Input: part model. Units: mm. Frame: model coordinates. A direction names the side the tool comes from. Round coordinates to 2 decimals unless told otherwise and drop trailing zeros. Loops run counter-clockwise (first coordinate to the right, second up) from the corner with the lowest first, then second, coordinate; pieces in that order, holes last.
(1) Cut plane B-B, the plane z = -8.5. Output: boundary loops of the cut face in (x, y), and give its area (3 significant figures).
(2) Line query: line 1 (Z direction, x = 4.15, y = 0); line 2 (Y direction, x = 4.2, z = -8.5); line 3 (Z direction, x = 3.25, y = 1). Output: solid intervals per line, ascending.
(3) Cut plane A-A, the plane x = -3.25. Output: boundary loops of the cut face in (y, z).
(4) First-contact query: pin 1 Ø6 at (x, y) = (3, -8) entering from -Z; pin 2 Ø1.5 at (x, y) = (0, 0.5) entering from +Z; pin 3 Ø4 at (y, z) = (-33.5, -1) entering from -X; pin 4 Ø1 at (y, z) = (-41, 4.5) entering from +X. Flat tips, straight axial feed; report the tip coordinate or a pass-through.
(5) Cut plane D-D, the plane z = 0. Output: boundary loops of the cut face in (x, y).
(6) Access query for faces 1 (the face through (-1, -3.5, -2.5)), 2 (the face through (5, 0, 0)), 3 (the face through (1.5, -2, 9)). Directions: +Z, -Z, +X, -X, +Y, -Y. A direction counts if a zero-diameter tool reaches every point of the face in a straight line with its end or side. Return the directions, or none.
(7) Cut plane C-C, the plane y = 0. Output: boundary loops of the cut face in (x, z), and give its area (3 significant figures).
(8) Draft query along X for faces 4 (the face through (-5, 0, 0)), 5 (the face through (-1.5, -2, -8)), 6 (the face through (3.27, -2.93, 11.9)). Return one class per face: released by +X, released by -X, zero draft, split by the parting line, or undercut.
from build123d import *

# Parameters (mm, degrees)
CROQUIS1_R                 = 2.5
SALIENTE_EXTRUIR1_DEPTH    = 50
CROQUIS2_R                 = 1.5
SALIENTE_EXTRUIR2_DEPTH    = 5
CORTAR_EXTRUIR1_DEPTH      = 56.167925464
CORTAR_EXTRUIR1_DEPTH_BACK = 56.167925464
CROQUIS3_W                 = 3
CROQUIS3_H                 = 8


with BuildPart() as part:
    # Croquis1 → Saliente-Extruir1 (new body)
    with BuildSketch(Plane(origin=(0, 0, 0), x_dir=(1, 0, 0), z_dir=(0, 1, 0))):
        with Locations(Location((0, 0, 0), (0, 0, 270))):
            Circle(CROQUIS1_R)
    extrude(amount=-SALIENTE_EXTRUIR1_DEPTH)

    # Croquis2 → Saliente-Extruir2 (add, symmetric)
    with BuildSketch(Plane(origin=(0, 0, 0), x_dir=(0, 0, -1), z_dir=(1, 0, 0))):
        with BuildLine():
            Line((10.5, -3.5), (-10.5, -3.5))
            ThreePointArc((-10.5, -3.5), (-11.914213562, -2.914213562), (-12.5, -1.5))
            Line((-12.5, -1.5), (-12.5, 1.5))
            ThreePointArc((-12.5, 1.5), (-11.914213562, 2.914213562), (-10.5, 3.5))
            Line((-10.5, 3.5), (10.5, 3.5))
            ThreePointArc((10.5, 3.5), (11.914213562, 2.914213562), (12.5, 1.5))
            Line((12.5, 1.5), (12.5, -1.5))
            ThreePointArc((12.5, -1.5), (11.914213562, -2.914213562), (10.5, -3.5))
        make_face()
        with Locations((-8.5, 0)):
            Circle(CROQUIS2_R, mode=Mode.SUBTRACT)
        with Locations((8.5, 0)):
            Circle(CROQUIS2_R, mode=Mode.SUBTRACT)
    extrude(amount=SALIENTE_EXTRUIR2_DEPTH, both=True)

    # Croquis3 → Cortar-Extruir1 (cut, two sides: drawn at the far end of the back side and taken through both)
    with BuildSketch(Plane(origin=(0, 3.5, 0), x_dir=(1, 0, 0), z_dir=(0, 1, 0)).offset(-CORTAR_EXTRUIR1_DEPTH_BACK)):
        with Locations((0, 8.5)):
            Rectangle(CROQUIS3_W, CROQUIS3_H)
        with Locations((0, -8.5)):
            Rectangle(CROQUIS3_W, CROQUIS3_H)
    extrude(amount=CORTAR_EXTRUIR1_DEPTH + CORTAR_EXTRUIR1_DEPTH_BACK, mode=Mode.SUBTRACT)


solid = part.part
Reported:
1. outline: (-5, -3.5) - (-1.5, -3.5) - (-1.5, -1.5) - (-5, -1.5) - close; (-5, 1.5) - (-1.5, 1.5) - (-1.5, 3.5) - (-5, 3.5) - close; (1.5, -3.5) - (5, -3.5) - (5, -1.5) - (1.5, -1.5) - close; (1.5, 1.5) - (5, 1.5) - (5, 3.5) - (1.5, 3.5) - close
1. area: 28.0 mm2
2. line 1: z = -12.5 to -10, -7 to 7, 10 to 12.5
2. line 2: y = -3.5 to -1.5, 1.5 to 3.5
2. line 3: z = -12.5 to -9.62, -7.38 to 7.38, 9.62 to 12.5
3. outline: (-3.5, -10.5) arc R2 ccw to (-1.5, -12.5) - (1.5, -12.5) arc R2 ccw to (3.5, -10.5) - (3.5, 10.5) arc R2 ccw to (1.5, 12.5) - (-1.5, 12.5) arc R2 ccw to (-3.5, 10.5) - close; hole circle Ø3 at (0, -8.5); hole circle Ø3 at (0, 8.5)
4. pin 1: stops at z = -2.5
4. pin 2: stops at z = 4.5
4. pin 3: stops at x = -2.5
4. pin 4: passes through
5. outline: (-5, -3.5) - (-2.5, -3.5) - (-2.5, -50) - (2.5, -50) - (2.5, -3.5) - (5, -3.5) - (5, 3.5) - (-5, 3.5) - close
6. face 1: -Y
6. face 2: +Z, -Z, +X, +Y, -Y
6. face 3: +Z, +Y, -Y
7. outline: (-5, -12.5) - (-1.5, -12.5) - (-1.5, -10) - (-5, -10) - close; (-5, -7) - (-1.5, -7) - (-1.5, -4.5) - (1.5, -4.5) - (1.5, -7) - (5, -7) - (5, 7) - (1.5, 7) - (1.5, 4.5) - (-1.5, 4.5) - (-1.5, 7) - (-5, 7) - close; (-5, 10) - (-1.5, 10) - (-1.5, 12.5) - (-5, 12.5) - close; (1.5, -12.5) - (5, -12.5) - (5, -10) - (1.5, -10) - close; (1.5, 10) - (5, 10) - (5, 12.5) - (1.5, 12.5) - close
7. area: 160 mm2
8. face 4: released by -X
8. face 5: undercut
8. face 6: zero draft
